Here's how the part is built. I have some questions about the finished solid (model axes, mm). A direction names the side the tool comes from. Coordinates: 2 decimals unless noted, no trailing zeros. Loops run counter-clockwise (first coordinate to the right, second up) from the corner with the lowest first, then second, coordinate; pieces in that order, holes last. Notation, with made-up numbers: (52, -29.75) -> (76, -29.75) arc R23 cw to (76, -2.75) -> close; hole circle Ø3 at (-9.75, 4.25). An arc over 180 degrees is marked (long way). Answer as a JSON object with one key per item and string values. Group by question number.
Q1. I'm going to push flat-ended pins straight in: pin 1 (2 mm diameter, centred on y = 1, z = 8.5, fed in from +X); pin 2 (1 mm diameter, centred on y = 2.5, z = 3, fed in from -X); pin 3 (3 mm diameter, centred on y = -4.5, z = 6.5, fed in from -X); pin 4 (2 mm diameter, centred on x = 3, z = 5, fed in from +Y) (1 decimal). Where does each tip first touch, or does it pass through?
Q2. Thinking about a two-plate mould opening in Z: for faces 6 (the cylindrical face through (3.38, -1.01, 6.71)), 7 (the flat face through (9.5, -5, 5)), 8 (the flat face through (7.8, -1.5, 10)), which applies, released by +Z, released by -Z, zero draft, split by the parting line, or undercut?
Q3. On a 3-axis mill with a long thin cutter (end or side, diameter ignored), from which of +Z, -Z, +X, -X, +Y, -Y can I reach the whole of each face in a straight line? I mean faces 1 (the flat face through (11, -9, 5)), 2 (the flat face through (8, -9, 5)), 3 (the cylindrical face through (9.215, -7.603, 5.07)), 4 (the flat face through (10.809, -2, 5)), 5 (the flat face through (5, 0, 5)). Say none if no direction works.
Q4. I want a section at A-A on x = 3. Write out the boundary of the cut face in (y, z), then the cut area to 3 significant figures.
Q5. I want a section at B-B on z = 5. Write out the boundary of the cut face in (x, y), then the cut area to 3 significant figures.
Q6. I want a section at C-C on x = 7. Write out the boundary of the cut face in (y, z), then the cut area to 3 significant figures.
Q7. I want a section at D-D on z = 1. Write out the boundary of the cut face in (x, y), then the cut area to 3 significant figures.
Q8. I need wall thicknesses on line 1 (Z direction, x = 3, y = -0.45); line 2 (Y direction, x = 8, z = 7.5); line 3 (X direction, y = -1.05, z = 5). Which ranges of each line are inside material? Lowest first, please.
```python
from build123d import *

# Parameters (mm, degrees)
BOSS_EXTRUDE1_DEPTH  = 10
M3_CLEARANCE_HOLE1_D = 3.5
CUT_EXTRUDE1_DEPTH   = 10
CUT_EXTRUDE2_START   = -10
CUT_EXTRUDE2_DEPTH   = 10


with BuildPart() as part:
    # Sketch1 → Boss-Extrude1 (new body)
    with BuildSketch(Plane.XY):
        with BuildLine():
            Line((0, 0), (8, 0))
            Line((8, 0), (8.5, 0))
            ThreePointArc((8.5, 0), (8.853553391, 0.146446609), (9, 0.5))
            Line((9, 0.5), (9, 3.5))
            ThreePointArc((9, 3.5), (9.146446609, 3.853553391), (9.5, 4))
            Line((9.5, 4), (10.309420257, 4))
            ThreePointArc((10.309420257, 4), (10.662973647, 3.853553391), (10.809420257, 3.5))
            Line((10.809420257, 3.5), (10.809420257, -7.604196011))
            ThreePointArc((10.809420257, -7.604196011), (10.897288222, -7.816328045), (11.109420257, -7.904196011))
            Line((11.109420257, -7.904196011), (11.7, -7.904196011))
            ThreePointArc((11.7, -7.904196011), (11.912132034, -7.992063976), (12, -8.204196011))
            Line((12, -8.204196011), (12, -8.7))
            ThreePointArc((12, -8.7), (11.912132034, -8.912132034), (11.7, -9))
            Line((11.7, -9), (10.1244998, -9))
            ThreePointArc((10.1244998, -9), (9.5, -9.1), (8.8755002, -9))
            Line((8.8755002, -9), (6.3, -9))
            ThreePointArc((6.3, -9), (6.087867966, -8.912132034), (6, -8.7))
            Line((6, -8.7), (6, -8.2))
            ThreePointArc((6, -8.2), (6.070871215, -8.006350833), (6.25, -7.904196011))
            ThreePointArc((6.25, -7.904196011), (6.429128785, -7.802041189), (6.5, -7.608392022))
            Line((6.5, -7.608392022), (6.5, -2.2))
            ThreePointArc((6.5, -2.2), (6.441421356, -2.058578644), (6.3, -2))
            Line((6.3, -2), (0, -2))
            Line((0, -2), (0, 0))
        make_face()
    extrude(amount=BOSS_EXTRUDE1_DEPTH)

    # M3 Clearance Hole1 (through all)
    with Locations(Plane(origin=(0, 0, 0), x_dir=(1, 0, 0), z_dir=(0, 1, 0))):
        with Locations((3, -5)):
            Hole(M3_CLEARANCE_HOLE1_D / 2)

    # Sketch4 → Cut-Extrude1 (cut)
    with BuildSketch(Plane.XY.offset(10)):
        with BuildLine():
            Line((5.764081335, -2), (8.5, -2))
            ThreePointArc((8.5, -2), (9.207106781, -2.292893219), (9.5, -3))
            Line((9.5, -3), (9.5, -6.904196011))
            ThreePointArc((9.5, -6.904196011), (9.207106781, -7.611302792), (8.5, -7.904196011))
            Line((8.5, -7.904196011), (5.764081335, -7.904196011))
            Line((5.764081335, -7.904196011), (5.764081335, -2))
        make_face()
    extrude(amount=-CUT_EXTRUDE1_DEPTH, mode=Mode.SUBTRACT)

    # Sketch6 → Cut-Extrude2 (cut)
    with BuildSketch(Plane.XY.offset(10).offset(CUT_EXTRUDE2_START)):
        with BuildLine():
            Line((6.4, -8.2), (6.4, -8.7))
            ThreePointArc((6.4, -8.7), (6.487867966, -8.912132034), (6.7, -9))
            Line((6.7, -9), (6.3, -9))
            ThreePointArc((6.3, -9), (6.087867966, -8.912132034), (6, -8.7))
            Line((6, -8.7), (6, -8.2))
            ThreePointArc((6, -8.2), (6.070871215, -8.006350833), (6.25, -7.904196011))
            Line((6.25, -7.904196011), (6.695803989, -7.904196011))
            ThreePointArc((6.695803989, -7.904196011), (6.486638983, -7.990834993), (6.4, -8.2))
        make_face()
    extrude(amount=CUT_EXTRUDE2_DEPTH, mode=Mode.SUBTRACT)


solid = part.part
```
Result set:
{
 "1": {"pin 1": "stops at x = 10.81", "pin 2": "stops at x = 9", "pin 3": "stops at x = 9.5", "pin 4": "passes through"},
 "2": {"face 6": "undercut", "face 7": "zero draft", "face 8": "released by +Z"},
 "3": {"face 1": "+Z, -Z, +X, -Y", "face 2": "+Z, -Z, -X, -Y", "face 3": "+Z, -Z, -X", "face 4": "+Z, -Z, +X, +Y", "face 5": "+Z, -Z, -X, +Y"},
 "4": {"outline": "(-2, 0) -> (0, 0) -> (0, 3.25) -> (-2, 3.25) -> close; (-2, 6.75) -> (0, 6.75) -> (0, 10) -> (-2, 10) -> close", "area": "13.0 mm²"},
 "5": {"outline": "(0, -2) -> (1.25, -2) -> (1.25, 0) -> (0, 0) -> close; (4.75, -2) -> (8.5, -2) arc R1 cw to (9.5, -3) -> (9.5, -6.9) arc R1 cw to (8.5, -7.9) -> (6.7, -7.9) arc R0.3 ccw to (6.4, -8.2) -> (6.4, -8.7) arc R0.3 ccw to (6.7, -9) -> (8.88, -9) arc R2 ccw to (10.12, -9) -> (11.7, -9) arc R0.3 ccw to (12, -8.7) -> (12, -8.2) arc R0.3 ccw to (11.7, -7.9) -> (11.11, -7.9) arc R0.3 cw to (10.81, -7.6) -> (10.81, 3.5) arc R0.5 ccw to (10.31, 4) -> (9.5, 4) arc R0.5 ccw to (9, 3.5) -> (9, 0.5) arc R0.5 cw to (8.5, 0) -> (4.75, 0) -> close", "area": "36.1 mm²"},
 "6": {"outline": "(-9, 0) -> (-7.9, 0) -> (-7.9, 10) -> (-9, 10) -> close; (-2, 0) -> (0, 0) -> (0, 10) -> (-2, 10) -> close", "area": "31.0 mm²"},
 "7": {"outline": "(0, -2) -> (8.5, -2) arc R1 cw to (9.5, -3) -> (9.5, -6.9) arc R1 cw to (8.5, -7.9) -> (6.7, -7.9) arc R0.3 ccw to (6.4, -8.2) -> (6.4, -8.7) arc R0.3 ccw to (6.7, -9) -> (8.88, -9) arc R2 ccw to (10.12, -9) -> (11.7, -9) arc R0.3 ccw to (12, -8.7) -> (12, -8.2) arc R0.3 ccw to (11.7, -7.9) -> (11.11, -7.9) arc R0.3 cw to (10.81, -7.6) -> (10.81, 3.5) arc R0.5 ccw to (10.31, 4) -> (9.5, 4) arc R0.5 ccw to (9, 3.5) -> (9, 0.5) arc R0.5 cw to (8.5, 0) -> (0, 0) -> close", "area": "43.1 mm²"},
 "8": {"line 1": "z = 0 to 3.25, 6.75 to 10", "line 2": "y = -9 to -7.9, -2 to 0", "line 3": "x = 0 to 1.25, 4.75 to 10.81"}
}
